Autodesk Inventor part; units mm, degrees
ref_plane "YZ Plane" through (0, 0, 0) normal (1, 0, 0) x (0, 1, 0)
ref_plane "XZ Plane" through (0, 0, 0) normal (0, 1, 0) x (-1, 0, 0)
ref_plane "XY Plane" through (0, 0, 0) normal (0, 0, 1) x (1, 0, 0)
sketch "Sketch1" plane through (0, 0, 0) normal (0, 1, 0) x (-1, 0, 0)
  line L0 (0, 0) -> (-30, 0)
  line L1 (-30, 0) -> (-30, 20)
  line L2 (-30, 20) -> (-115, 20)
  line L3 (-115, 20) -> (-115, 0)
  line L4 (-115, 0) -> (-145, 0)
  line L5 (0, 3) -> (-27, 3)
  line L6 (-27, 3) -> (-27, 23)
  line L7 (-27, 23) -> (-118, 23)
  line L8 (-118, 23) -> (-118, 3)
  line L9 (-118, 3) -> (-145, 3)
  line L10 (0, 0) -> (0, 3)
  line L11 (-145, 0) -> (-145, 3)
  dimension "d0" = 30
  dimension "d1" = 20
  dimension "d2" = 3
  dimension "d28" = 85
extrude "Extrusion1" add sketch "Sketch1" along normal blind 82
sketch "Sketch2" plane through (27, 0, 23) normal (0, 0, 1) x (1, 0, 0)
  line L0 (0, 82) -> (91, 82)
  line L1 (45.5, 82) -> (45.5, 0) construction
  line L2 (0, 0) -> (91, 0)
  circle A0 centre (45.5, 41) radius 32.5 construction
  line L3 (45.5, 41) -> (68.481, 63.981) construction
  circle A1 centre (68.481, 63.981) radius 3.05
  circle A2 centre (22.519, 63.981) radius 3.05
  circle A3 centre (22.519, 18.019) radius 3.05
  circle A4 centre (68.481, 18.019) radius 3.05
  circle A5 centre (45.5, 41) radius 25.0125
  point P0 (-27, 0)
  dimension "d6" = 65
  dimension "d7" = 6.1
  dimension "d8" = 45
  dimension "d11" = 360
  dimension "d15" = 50.025
extrude "Extrusion2" cut sketch "Sketch2" against normal blind 82
sketch "Sketch3" plane through (0, 0, 3) normal (0, 0, 1) x (1, 0, 0)
  circle A0 centre (72.5, 41) radius 25.0125 construction
  line L0 (12.5, 66) -> (132.5, 66) construction
  line L1 (132.5, 66) -> (132.5, 16) construction
  line L2 (132.5, 16) -> (12.5, 16) construction
  line L3 (12.5, 16) -> (12.5, 66) construction
  line L4 (12.5, 66) -> (132.5, 16) construction
  line L5 (132.5, 66) -> (12.5, 16) construction
  circle A1 centre (12.5, 66) radius 3.05
  circle A2 centre (12.5, 16) radius 3.05
  circle A3 centre (132.5, 66) radius 3.05
  circle A4 centre (132.5, 16) radius 3.05
  dimension "d29" = 6.1
  dimension "d30" = 120
  dimension "d31" = 50
extrude "Extrusion3" cut sketch "Sketch3" against normal blind 10
properties part number "MotorBracket"
Work out the finished part from the listing and answer in its coordinate system (mm). A direction names the side the tool comes from. Round coordinates to 2 decimals unless told otherwise and drop trailing zeros. Write each loop counter-clockwise with the first axis right and the second up, starting at its lowest first coordinate (ties: lowest second). Pieces come first, ordered by that corner, then holes.
1) A tool of negligible diameter and unlimited length cuts with its end or side. For faces 4 (the flat face through (118, 40, 13)), 5 (the flat face through (13, 40, 3)), 6 (the flat face through (30, 40, 10)), from which of +Z, -Z, +X, -X, +Y, -Y can it reach the whole face along a straight path? Write none if from no direction.
2) A cutting plane is placed at A-A (x = 132.5). Give the vertices of the cut face in (y, z), plus the area to 3 significant figures.
3) The mould has two halves that part along X. Classify faces 1 (the flat face through (15, 40, 0)), 2 (the cylindrical face through (10.25, 18.06, 1.52)), 3 (the flat face through (145, 40, 1)): pulls with the +X half, pulls with the -X half, needs draft (parallel to the pull), parting line crosses it, or undercut.
4) Straight lines are drawn through the part: line 1 (Y direction, x = 12.5, z = 1.6); line 2 (X direction, y = 71, z = 2); line 3 (X direction, y = 59.5, z = 11). For each, find the intervals that lie inside material, in ascending order.
5) A cutting plane is placed at C-C (x = 72.5). Give the vertices of the cut face in (y, z), plus the area to 3 significant figures.
6) Given pin 1 Ø3.5 at (x, y) = (132.5, 16) entering from +Z; pin 2 Ø1.5 at (y, z) = (37, 5) entering from +X; pin 3 Ø10 at (y, z) = (47, 15) entering from -X; pin 4 Ø2 at (x, y) = (101.5, 35.5) entering from -Z, each flat-ended and moving along its own axis, determine where each tip first touches the part or whether it passes through.
7) A cutting plane is placed at B-B (y = 41). Give the vertices of the cut face in (x, z).
8) A cutting plane is placed at D-D (z = 15). Give the vertices of the cut face in (x, y), plus the area to 3 significant figures.
Completed:
1. face 4: +Z, +X, +Y, -Y
1. face 5: +Z, -X, +Y, -Y
1. face 6: -Z, +Y, -Y
2. outline: (0, 0) - (12.95, 0) - (12.95, 3) - (0, 3) - close; (19.05, 0) - (62.95, 0) - (62.95, 3) - (19.05, 3) - close; (69.05, 0) - (82, 0) - (82, 3) - (69.05, 3) - close
2. area: 209 mm2
3. face 1: needs draft
3. face 2: undercut
3. face 3: pulls with the +X half
4. line 1: y = 0 to 12.95, 19.05 to 62.95, 69.05 to 82
4. line 2: x = 0 to 30, 115 to 145
4. line 3: x = 27 to 30, 115 to 118
5. outline: (0, 20) - (15.99, 20) - (15.99, 23) - (0, 23) - close; (66.01, 20) - (82, 20) - (82, 23) - (66.01, 23) - close
5. area: 95.9 mm2
6. pin 1: passes through
6. pin 2: stops at x = 118
6. pin 3: stops at x = 27
6. pin 4: stops at z = 20
7. outline: (0, 0) - (30, 0) - (30, 20) - (47.49, 20) - (47.49, 23) - (27, 23) - (27, 3) - (0, 3) - close; (97.51, 20) - (115, 20) - (115, 0) - (145, 0) - (145, 3) - (118, 3) - (118, 23) - (97.51, 23) - close
8. outline: (27, 0) - (30, 0) - (30, 82) - (27, 82) - close; (115, 0) - (118, 0) - (118, 82) - (115, 82) - close
8. area: 492 mm2
